```python
from build123d import *

# Parameters (mm, degrees)
F1_DEPTH = 304.8
F2_R     = 3.175
F3_DEPTH = 25.4
F4_R     = 1.5875
F5_DEPTH = 25.4


with BuildPart() as f1:
    # F0 (on Front) → F1 (new body)
    with BuildSketch(Plane.XZ):
        Polygon((-9.525, 12.7), (-12.7, 12.7), (-12.7, -12.7), (12.7, -12.7), (12.7, 12.7), (9.525, 12.7), (9.525, -9.525), (-9.525, -9.525), align=None)
    extrude(amount=-F1_DEPTH)

    # F2 (on face) → F3 (cut, through all)
    with BuildSketch(Plane.YZ.offset(12.7)):
        with Locations((260.35, -4.7498)):
            Circle(F2_R)
    extrude(amount=-F3_DEPTH, mode=Mode.SUBTRACT)

    # F4 (on face) → F5 (cut)
    with BuildSketch(Plane(origin=(0, 0, -12.7), x_dir=(1, 0, 0), z_dir=(0, 0, -1))):
        with Locations((0, -19.05)):
            Circle(F4_R)
        with Locations((0, -95.25)):
            Circle(F4_R)
        with Locations((0, -171.45)):
            Circle(F4_R)
    extrude(amount=-F5_DEPTH, mode=Mode.SUBTRACT)


solid = f1.part
```
Geometry: final body of the model. Coordinates: model frame, mm. A direction names the side the tool comes from. Round coordinates to 2 decimals unless told otherwise and drop trailing zeros. Order: outer loops, then holes, each group sorted by start corner. A loop starts at its lowest first (then second) coordinate and runs counter-clockwise, first axis right, second up. Notation, with made-up numbers: (75.5, 66) -> (128.5, 66) arc R10 ccw to (128.5, 71) -> close; hole circle Ø2 at (83, 14.5). An arc over 180 degrees is marked (long way). Write each question's results on one line, items separated by ' | '.
Q1. Ray query, line 1 along Y through (x, z) = (0, -12.1); line 2 along Z through (x, y) = (11.55, 260.35); line 3 along X through (y, z) = (165, -3) (3 decimals). Return the intervals inside material, ascending.
Response values:
line 1: 0 to 17.46, 20.64 to 93.66, 96.84 to 169.86, 173.04 to 304.8 | line 2: -12.7 to -7.92, -1.57 to 12.7 | line 3: -12.7 to -9.525, 9.525 to 12.7
Q2. Pull-direction query (Z, two-part tool) for faces 3 (the face through (-11.09, 257.18, -4.61)), 4 (the face through (0, 0, -10)), 5 (the face through (0, 150, -9.525)); classes: released by +Z, released by -Z, zero draft, split by the parting line, or undercut.
Response values:
face 3: undercut | face 4: zero draft | face 5: released by +Z
Q3. Access query for faces 1 (the face through (-9.525, 150, 1)), 2 (the face through (0, 150, -12.7)). Directions: +Z, -Z, +X, -X, +Y, -Y. A direction counts if a zero-diameter tool reaches every point of the face in a straight line with its end or side. Return the directions, or none.
Response values:
face 1: +Z, +Y, -Y | face 2: -Z, +X, -X, +Y, -Y
Q4. Section query C-C (y = 100). Output: boundary loops of the cut face in (x, z) (3 decimals).
Response values:
outline: (-12.7, -12.7) -> (12.7, -12.7) -> (12.7, 12.7) -> (9.525, 12.7) -> (9.525, -9.525) -> (-9.525, -9.525) -> (-9.525, 12.7) -> (-12.7, 12.7) -> close
Q5. Section query A-A (y = 260.35). Output: boundary loops of the cut face in (x, z) (3 decimals), and give its area (3 significant figures).
Response values:
outline: (-12.7, -12.7) -> (12.7, -12.7) -> (12.7, -7.925) -> (9.525, -7.925) -> (9.525, -9.525) -> (-9.525, -9.525) -> (-9.525, -7.925) -> (-12.7, -7.925) -> close; (-12.7, -1.575) -> (-9.525, -1.575) -> (-9.525, 12.7) -> (-12.7, 12.7) -> close; (9.525, -1.575) -> (12.7, -1.575) -> (12.7, 12.7) -> (9.525, 12.7) -> close | area: 181 mm²
Q6. Section query B-B (z = 3.75). Output: boundary loops of the cut face in (x, y) (3 decimals), and give its area (3 significant figures).
Response values:
outline: (-12.7, 0) -> (-9.525, 0) -> (-9.525, 304.8) -> (-12.7, 304.8) -> close; (9.525, 0) -> (12.7, 0) -> (12.7, 304.8) -> (9.525, 304.8) -> close | area: 1,940 mm²
